Can you work these out from the drawing? Everything is in mm from the part's minimum corner. Round coordinates to 2 decimals unless told otherwise and drop trailing zeros. Write each loop counter-clockwise with the first axis right and the second up, starting at its lowest first coordinate (ties: lowest second). Pieces come first, ordered by that corner, then holes. Notation, with made-up numbers: (-19, -12) - (-11, -12) arc R22 cw to (-11, 7) - close; hole circle Ø5 at (72, -28). An arc over 180 degrees is marked (long way). One line per item, written item: value. Start each with the question number.
(1) I want a section at A-A on y = 13. List the corners of the cut face in (x, z) for me.
(2) I'm going to push flat-ended pins straight in: pin 1 Ø1.5 at (y, z) = (2, 1) entering from -X; pin 2 Ø0.9 at (y, z) = (22, 2) entering from +X; pin 3 Ø0.9 at (x, z) = (7.5, 1.5) entering from -Y. Where does each tip first touch, or does it pass through?
(3) I want a section at B-B on x = 14. List the corners of the cut face in (y, z) for me.
(4) I want a section at C-C on z = 1.65. List the corners of the cut face in (x, y) for me.
(5) I want a section at D-D on y = 22. List the corners of the cut face in (x, z) for me, plus the area to 3 significant figures.
(6) If I drill on L1, parallel to Y at x = 14, z = 1.95; L2, parallel to Y at x = 62.5, z = 2.3; L3, parallel to X at y = 11.5, z = 0.75, over which ranges is the centre line in solid material (lowest first)? Write a range as from..to.
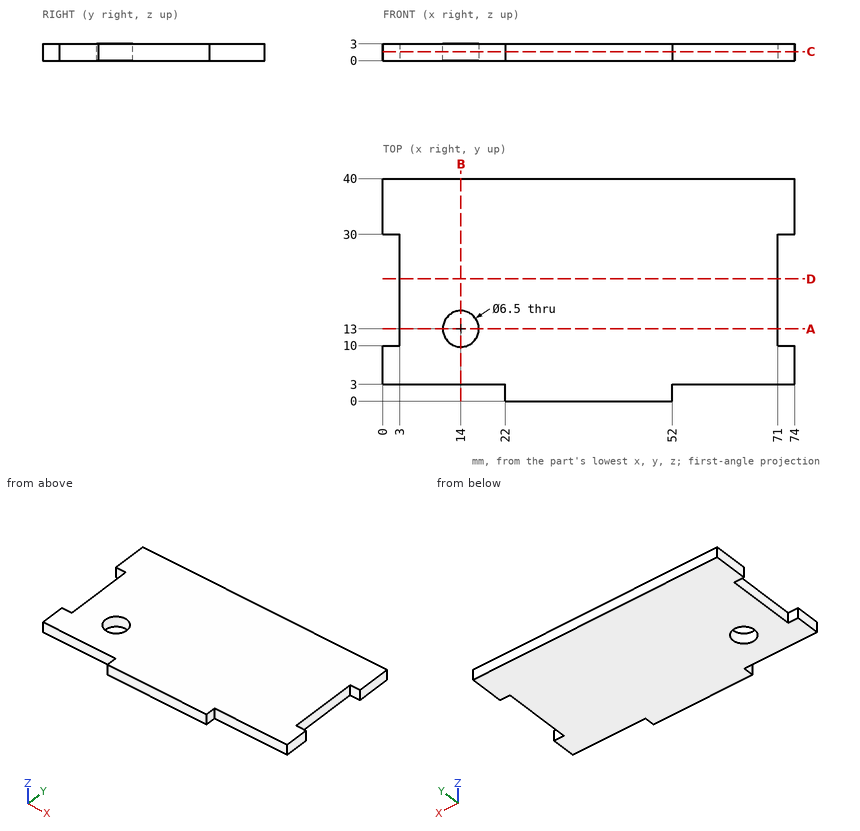
Established:
1. outline: (3, 0) - (10.75, 0) - (10.75, 3) - (3, 3) - close; (17.25, 0) - (71, 0) - (71, 3) - (17.25, 3) - close
2. pin 1: x = 22
2. pin 2: x = 71
2. pin 3: y = 3
3. outline: (3, 0) - (9.75, 0) - (9.75, 3) - (3, 3) - close; (16.25, 0) - (40, 0) - (40, 3) - (16.25, 3) - close
4. outline: (0, 3) - (22, 3) - (22, 0) - (52, 0) - (52, 3) - (74, 3) - (74, 10) - (71, 10) - (71, 30) - (74, 30) - (74, 40) - (0, 40) - (0, 30) - (3, 30) - (3, 10) - (0, 10) - close; hole circle Ø6.5 at (14, 13)
5. outline: (3, 0) - (71, 0) - (71, 3) - (3, 3) - close
5. area: 204 mm2
6. L1: 3..9.75, 16.25..40
6. L2: 3..40
6. L3: 3..11.12, 16.88..71
